Answer from the drawing. Dimensions are ordinates in mm from the lowest x, y and z of the part. Round coordinates to 2 decimals unless told otherwise and drop trailing zeros. Write each loop counter-clockwise with the first axis right and the second up, starting at its lowest first coordinate (ties: lowest second). Pieces come first, ordered by that corner, then holes.
1. Find section C-C (x = 1648). Write down the section's boundary in (y, z).
2. Find section B-B (z = 15). Write down the section's boundary in (x, y).
3. Find section A-A (y = 95). Write down the section's boundary in (x, z), and give its area (3 significant figures).
4. Straight lines are drawn through the part: probe 1 along X at (y, z) = (477, 27); probe 2 along Y at (x, z) = (150, 29). For each, find the intervals that lie inside material, in ascending order.
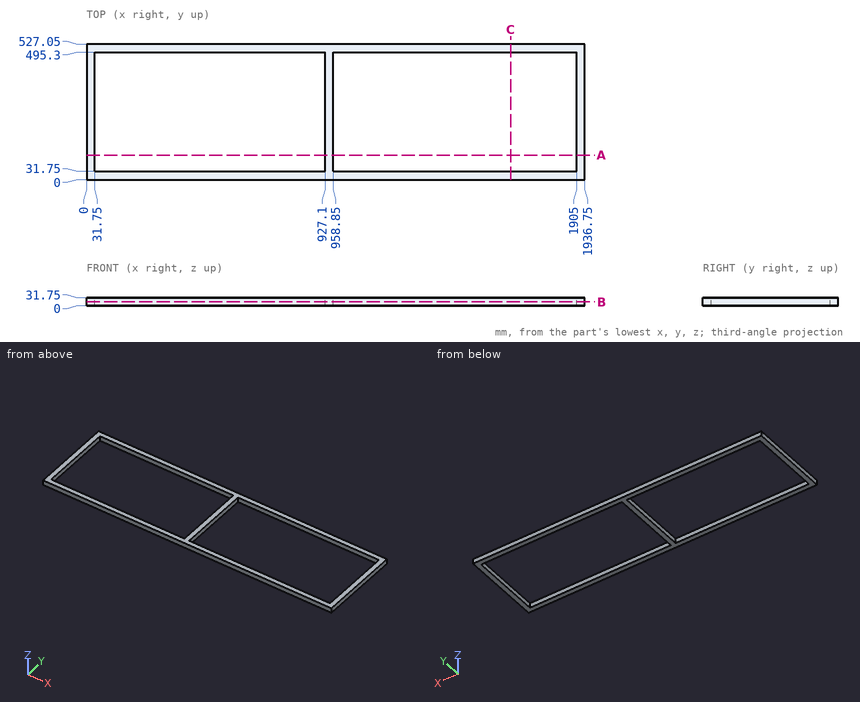
Worked answers:
1. outline: (0, 0) - (31.75, 0) - (31.75, 31.75) - (0, 31.75) - close; (495.3, 0) - (527.05, 0) - (527.05, 31.75) - (495.3, 31.75) - close
2. outline: (0, 0) - (1936.75, 0) - (1936.75, 527.05) - (0, 527.05) - close; hole (31.75, 31.75) - (927.1, 31.75) - (927.1, 495.3) - (31.75, 495.3) - close; hole (958.85, 31.75) - (1905, 31.75) - (1905, 495.3) - (958.85, 495.3) - close
3. outline: (0, 0) - (31.75, 0) - (31.75, 31.75) - (0, 31.75) - close; (927.1, 0) - (958.85, 0) - (958.85, 31.75) - (927.1, 31.75) - close; (1905, 0) - (1936.75, 0) - (1936.75, 31.75) - (1905, 31.75) - close
3. area: 3,020 mm2
4. probe 1: x = 0 to 31.75, 927.1 to 958.85, 1905 to 1936.75
4. probe 2: y = 0 to 31.75, 495.3 to 527.05
